Design review of the part built by this model. Coordinates are the model's own, in mm. A direction names the side the tool comes from. Coordinates: 2 decimals unless noted, no trailing zeros. Loops run counter-clockwise (first coordinate to the right, second up) from the corner with the lowest first, then second, coordinate; pieces in that order, holes last. Notation, with made-up numbers: (14, 35.25) -> (68, 35.25) arc R13 cw to (68, 42.25) -> close; hole circle Ø6 at (43.25, 53.5). An arc over 180 degrees is marked (long way). Use a Markdown table: item, result. Add a question column.
Q1. Take a section at B-B on x = -24. Write out the cut boundary in (y, z).
Q2. Take a section at C-C on y = -56.5. Write out the cut boundary in (x, z), plus the area to 3 significant figures.
Q3. Take a section at D-D on y = -30. Write out the cut boundary in (x, z), plus the area to 3 significant figures.
Q4. For probe 1 along X at (y, z) = (-45, 3.75); probe 2 along X at (y, z) = (-59, 8.5); probe 3 along X at (y, z) = (-30, 8.25), list the stretches that pass through material, from the lowest coordinate up.
Q5. For faces 1 (the face through (-1, -27, 10)), 2 (the face through (-35, -68, 5)), list the 3-axis set-ups (+Z, -Z, +X, -X, +Y, -Y) from which the entire face can be reached by the end or side of a thin tool; tool diameter is ignored.
Q6. Take a section at A-A on z = 2.75. Write out the cut boundary in (x, y).
Q7. Clearance check with a flat-ended pin moving along its axis: pin 1 Ø3 at (x, z) = (-2, 6.5) entering from -Y. State where the tip first meets the part, or that it passes through.
from build123d import *

# Parameters (mm, degrees)
F1_DEPTH = 10


with BuildPart() as f1:
    # F0 (on Top) → F1 (new body)
    with BuildSketch(Plane.XY):
        with BuildLine():
            Line((45, 0), (0, 0))
            Line((0, 0), (0, -35))
            Line((0, -35), (5, -35))
            Line((5, -35), (11.0542490694, -35))
            ThreePointArc((11.0542490694, -35), (21.1660409917, -25.4925456214), (35, -24.3693346885))
            Line((35, -24.3693346885), (35, -20))
            Line((35, -20), (45, -20))
            Line((45, -20), (45, 0))
        make_face()
        with BuildLine():
            Line((0, -35), (0, 0))
            Line((0, 0), (-45, 0))
            Line((-45, 0), (-45, -20))
            Line((-45, -20), (-35, -20))
            Line((-35, -20), (-35, -24.3693346885))
            ThreePointArc((-35, -24.3693346885), (-21.1660409917, -25.4925456214), (-11.0542490694, -35))
            Line((-11.0542490694, -35), (-5, -35))
            Line((-5, -35), (0, -35))
        make_face()
        Polygon((65, -20), (45, 0), (45, -20), align=None)
        Polygon((-45, -20), (-45, 0), (-65, -20), align=None)
        with BuildLine():
            Line((65, -20), (45, -20))
            Line((45, -20), (45, -30.3156087011))
            ThreePointArc((45, -30.3156087011), (49.2135509862, -36.9586799562), (50.6869892627, -44.6861237288))
            ThreePointArc((50.6869892627, -44.6861237288), (46.3088607801, -57.5201950726), (35, -65.002912769))
            Line((35, -65.002912769), (35, -70))
            Line((35, -70), (65, -70))
            Line((65, -70), (65, -20))
        make_face()
        with BuildLine():
            Line((45, -30.3156087011), (45, -20))
            Line((45, -20), (35, -20))
            Line((35, -20), (35, -24.3693346885))
            ThreePointArc((35, -24.3693346885), (40.420009999, -26.6361302142), (45, -30.3156087011))
        make_face()
        with BuildLine():
            Line((11.0542490694, -35), (5, -35))
            Line((5, -35), (9.3708041453, -39.3708041453))
            ThreePointArc((9.3708041453, -39.3708041453), (10.0902885727, -37.1383212628), (11.0542490694, -35))
        make_face()
        with BuildLine():
            Line((-9.3708041453, -39.3708041453), (-5, -35))
            Line((-5, -35), (-11.0542490694, -35))
            ThreePointArc((-11.0542490694, -35), (-10.0902885727, -37.1383212628), (-9.3708041453, -39.3708041453))
        make_face()
        with BuildLine():
            Line((-35, -20), (-45, -20))
            Line((-45, -20), (-45, -30.3156087011))
            ThreePointArc((-45, -30.3156087011), (-40.420009999, -26.6361302142), (-35, -24.3693346885))
            Line((-35, -24.3693346885), (-35, -20))
        make_face()
        with BuildLine():
            Line((-45, -30.3156087011), (-45, -20))
            Line((-45, -20), (-65, -20))
            Line((-65, -20), (-65, -70))
            Line((-65, -70), (-35, -70))
            Line((-35, -70), (-35, -65.002912769))
            ThreePointArc((-35, -65.002912769), (-49.8652066354, -50.5033003341), (-45, -30.3156087011))
        make_face()
        with BuildLine():
            ThreePointArc((50.6869892627, -44.6861237288), (49.2135509862, -36.9586799562), (45, -30.3156087011))
            Line((45, -30.3156087011), (45, -35))
            Line((45, -35), (44.2619337604, -35))
            ThreePointArc((44.2619337604, -35), (46.439773042, -39.6270491449), (47.1869892627, -44.6861237288))
            ThreePointArc((47.1869892627, -44.6861237288), (43.815465612, -55.0126021241), (35, -61.3601129606))
            Line((35, -61.3601129606), (35, -65))
            Line((35, -65), (35, -65.002912769))
            ThreePointArc((35, -65.002912769), (46.3088607801, -57.5201950726), (50.6869892627, -44.6861237288))
        make_face()
        with BuildLine():
            Line((45, -35), (45, -30.3156087011))
            ThreePointArc((45, -30.3156087011), (40.420009999, -26.6361302142), (35, -24.3693346885))
            Line((35, -24.3693346885), (35, -28.0121344969))
            ThreePointArc((35, -28.0121344969), (40.2269255495, -30.7161651365), (44.2619337604, -35))
            Line((44.2619337604, -35), (45, -35))
        make_face()
        with BuildLine():
            ThreePointArc((35, -24.3693346885), (21.1660409917, -25.4925456214), (11.0542490694, -35))
            Line((11.0542490694, -35), (15.112044765, -35))
            ThreePointArc((15.112044765, -35), (23.8858324541, -28.1756246545), (35, -28.0121344969))
            Line((35, -28.0121344969), (35, -24.3693346885))
        make_face()
        with BuildLine():
            Line((15.112044765, -35), (11.0542490694, -35))
            ThreePointArc((11.0542490694, -35), (10.0902885727, -37.1383212628), (9.3708041453, -39.3708041453))
            Line((9.3708041453, -39.3708041453), (12.344376437, -42.344376437))
            ThreePointArc((12.344376437, -42.344376437), (13.311166148, -38.5150284196), (15.112044765, -35))
        make_face()
        with BuildLine():
            Line((12.344376437, -42.344376437), (9.3708041453, -39.3708041453))
            ThreePointArc((9.3708041453, -39.3708041453), (14.8369031184, -59.5345223463), (35, -65.002912769))
            Line((35, -65.002912769), (35, -65))
            Line((35, -65), (32.0287365544, -62.0287365544))
            ThreePointArc((32.0287365544, -62.0287365544), (17.3126205919, -57.0604923995), (12.344376437, -42.344376437))
        make_face()
        with BuildLine():
            Line((-12.344376437, -42.344376437), (-9.3708041453, -39.3708041453))
            ThreePointArc((-9.3708041453, -39.3708041453), (-10.0902885727, -37.1383212628), (-11.0542490694, -35))
            Line((-11.0542490694, -35), (-15.112044765, -35))
            ThreePointArc((-15.112044765, -35), (-13.311166148, -38.5150284196), (-12.344376437, -42.344376437))
        make_face()
        with BuildLine():
            ThreePointArc((-8.6869892627, -44.6861237288), (-8.8586445437, -42.006561028), (-9.3708041453, -39.3708041453))
            Line((-9.3708041453, -39.3708041453), (-12.344376437, -42.344376437))
            ThreePointArc((-12.344376437, -42.344376437), (-12.2263803894, -43.5126085924), (-12.1869892627, -44.6861237288))
            ThreePointArc((-12.1869892627, -44.6861237288), (-18.1702748355, -57.8624391774), (-32.0287365544, -62.0287365544))
            Line((-32.0287365544, -62.0287365544), (-35, -65))
            Line((-35, -65), (-35, -65.002912769))
            ThreePointArc((-35, -65.002912769), (-16.8529179189, -61.3079952462), (-8.6869892627, -44.6861237288))
        make_face()
        with BuildLine():
            Line((-15.112044765, -35), (-11.0542490694, -35))
            ThreePointArc((-11.0542490694, -35), (-21.1660409917, -25.4925456214), (-35, -24.3693346885))
            Line((-35, -24.3693346885), (-35, -28.0121344969))
            ThreePointArc((-35, -28.0121344969), (-23.8858324541, -28.1756246545), (-15.112044765, -35))
        make_face()
        with BuildLine():
            ThreePointArc((-35, -24.3693346885), (-40.420009999, -26.6361302142), (-45, -30.3156087011))
            Line((-45, -30.3156087011), (-45, -35))
            Line((-45, -35), (-44.2619337604, -35))
            ThreePointArc((-44.2619337604, -35), (-40.2269255495, -30.7161651365), (-35, -28.0121344969))
            Line((-35, -28.0121344969), (-35, -24.3693346885))
        make_face()
        with BuildLine():
            Line((-45, -35), (-45, -30.3156087011))
            ThreePointArc((-45, -30.3156087011), (-49.8652066354, -50.5033003341), (-35, -65.002912769))
            Line((-35, -65.002912769), (-35, -65))
            Line((-35, -65), (-35, -61.3601129606))
            ThreePointArc((-35, -61.3601129606), (-46.197488337, -50.4872805374), (-44.2619337604, -35))
            Line((-44.2619337604, -35), (-45, -35))
        make_face()
        with BuildLine():
            ThreePointArc((35, -61.3601129606), (33.5289411752, -61.7591845411), (32.0287365544, -62.0287365544))
            Line((32.0287365544, -62.0287365544), (35, -65))
            Line((35, -65), (35, -61.3601129606))
        make_face()
        with BuildLine():
            Line((-35, -65), (-32.0287365544, -62.0287365544))
            ThreePointArc((-32.0287365544, -62.0287365544), (-33.5289411752, -61.7591845411), (-35, -61.3601129606))
            Line((-35, -61.3601129606), (-35, -65))
        make_face()
    extrude(amount=F1_DEPTH)


solid = f1.part
Answer list:
| question | item | result |
|---|---|---|
| 1 | outline | (-64.9, 0) -> (-61.24, 0) -> (-61.24, 10) -> (-64.9, 10) -> close; (-28.14, 0) -> (0, 0) -> (0, 10) -> (-28.14, 10) -> close |
| 2 | outline | (-65, 0) -> (-42.6, 0) -> (-42.6, 10) -> (-65, 10) -> close; (-16.78, 0) -> (-12.33, 0) -> (-12.33, 10) -> (-16.78, 10) -> close; (12.33, 0) -> (16.78, 0) -> (16.78, 10) -> (12.33, 10) -> close; (42.6, 0) -> (65, 0) -> (65, 10) -> (42.6, 10) -> close |
| 2 | area | 537 mm² |
| 3 | outline | (-65, 0) -> (-39.2, 0) -> (-39.2, 10) -> (-65, 10) -> close; (-20.17, 0) -> (20.17, 0) -> (20.17, 10) -> (-20.17, 10) -> close; (39.2, 0) -> (65, 0) -> (65, 10) -> (39.2, 10) -> close |
| 3 | area | 919 mm² |
| 4 | probe 1 | -65 to -47.18, -12.19 to -8.69, 8.69 to 12.19, 47.18 to 65 |
| 4 | probe 2 | -65 to -39.75, -19.62 to -14.32, 14.32 to 19.62, 39.75 to 65 |
| 4 | probe 3 | -65 to -39.2, -20.17 to 20.17, 39.2 to 65 |
| 5 | face 1 | +Z, +X, -X, +Y, -Y |
| 5 | face 2 | +Z, -Z, -Y |
| 6 | outline | (-65, -70) -> (-35, -70) -> (-35, -65) arc R21 ccw to (-9.37, -39.37) -> (-5, -35) -> (5, -35) -> (9.37, -39.37) arc R21 ccw to (35, -65) -> (35, -70) -> (65, -70) -> (65, -20) -> (45, 0) -> (-45, 0) -> (-65, -20) -> close; hole circle Ø35 at (-29.69, -44.69); hole circle Ø35 at (29.69, -44.69) |
| 7 | pin 1 | y = -35 |
